Autodesk Fusion 360 part; units mm, degrees
sketch "Sketch1" plane through (0, 0, 0) normal (0, 0, 1) x (1, 0, 0)
  circle A0 centre (0, 0) radius 20
  line L0 (1, -19.975) -> (1, -21.1)
  line L1 (1, -21.1) -> (-1, -21.1)
  line L2 (-1, -21.1) -> (-1, -19.975)
  line L3 (18.7731, 9.684) -> (17.7988, 9.1215)
  line L4 (17.7731, 11.416) -> (18.7731, 9.684)
  line L5 (16.7988, 10.8535) -> (17.7731, 11.416)
  line L6 (-17.7731, 11.416) -> (-16.7988, 10.8535)
  line L7 (-18.7731, 9.684) -> (-17.7731, 11.416)
  line L8 (-17.7988, 9.1215) -> (-18.7731, 9.684)
  dimension "d5" = 40
  dimension "d9" = 2
  dimension "d12" = 360
extrude "Extrude2" add sketch "Sketch1" along normal blind 30 contours A0
shell "Shell2" thickness 1.5 removed faces 1 at (-4.9181, 4.3771, 30)
extrude "Extrude3" add sketch "Sketch1" along normal up to surface (30 mm away) contours A0 L3 L4 L5 | A0 L0 L1 L2 | A0 L6 L7 L8
The model under review builds one solid part; all positions refer to its coordinate system, in mm. A direction names the side the tool comes from. Give positions to 0.01 mm unless a question says otherwise; leave off trailing zeros. Loops run counter-clockwise (first coordinate to the right, second up) from the corner with the lowest first, then second, coordinate; pieces in that order, holes last. Notation, with made-up numbers: (-28.75, 18.25) -> (-12.75, 18.25) arc R22 cw to (-12.75, 55.25) -> close; hole circle Ø6 at (-19.5, 82). An arc over 180 degrees is marked (long way). Write each question's results on one line, items separated by ' | '.
1) Tool access review of faces 1 (the face through (17.28, 11.13, 14.79)), 2 (the face through (-18.28, 9.4, 14.79)), 3 (the face through (-4.01, 18.06, 15.55)), 4 (the face through (1, -20.5, 14.8)), 5 (the face through (-1, -20.5, 14.8)): name each direction out of +Z, -Z, +X, -X, +Y, -Y from which nothing blocks a thin tool from reaching the whole face with its end or side.
Conclusion:
face 1: +Z, -Z, +Y | face 2: +Z, -Z, -X | face 3: +Z | face 4: +Z, -Z, +X, -Y | face 5: +Z, -Z, -X, -Y
2) Draft analysis for pull direction X (two halves, no side actions). For faces 6 (the face through (-17.18, -10.24, 14.79)), 7 (the face through (0, 0, 1.5)), 8 (the face through (18.293, 9.407, 14.79)), state which applies: pulls with the +X half, pulls with the -X half, needs draft (parallel to the pull), parting line crosses it, or undercut.
Conclusion:
face 6: pulls with the -X half | face 7: undercut | face 8: pulls with the +X half
3) Take a section at A-A, the plane y = 0. Give the boundary of the cut face in (x, z).
Conclusion:
outline: (-20, 0) -> (20, 0) -> (20, 30) -> (18.5, 30) -> (18.5, 1.5) -> (-18.5, 1.5) -> (-18.5, 30) -> (-20, 30) -> close
4) Take a section at C-C, the plane z = 8. Give the boundary of the cut face in (x, y) (1 decimal), plus the area to 3 significant figures.
Conclusion:
outline: (-18.8, 9.7) -> (-17.8, 9.1) arc R20 ccw to (-1, -20) -> (-1, -21.1) -> (1, -21.1) -> (1, -20) arc R20 ccw to (17.8, 9.1) -> (18.8, 9.7) -> (17.8, 11.4) -> (16.8, 10.9) arc R20 ccw to (-16.8, 10.9) -> (-17.8, 11.4) -> close; hole circle Ø37 at (0, 0) | area: 188 mm^2
5) Insertion check: pin 1 Ø12 at (y, z) = (13, 17.5) entering from +X; pin 2 Ø2 at (x, z) = (-3, 8.5) entering from +Y; pin 3 Ø1 at (x, z) = (-2, 25) entering from -Y; pin 4 Ø8 at (x, y) = (1.5, 1) entering from -Z. Each pin has a flat end and moves straight along its axis. Give the tip position at first contact, or say it passes through.
Conclusion:
pin 1: stops at x = 18.77 | pin 2: stops at y = 19.9 | pin 3: stops at y = -19.94 | pin 4: stops at z = 0
6) Take a section at B-B, the plane x = 0. Give the boundary of the cut face in (y, z), plus the area to 4 significant figures.
Conclusion:
outline: (-21.1, 0) -> (20, 0) -> (20, 30) -> (18.5, 30) -> (18.5, 1.5) -> (-18.5, 1.5) -> (-18.5, 30) -> (-21.1, 30) -> close | area: 178.5 mm^2
7) For line 1 along Y through (x, z) = (0, 9); line 2 along X through (y, z) = (0, 18.25); line 3 along Z through (x, y) = (-13, -0.5), list the stretches that pass through material, from the lowest coordinate up. Write a range as from..to.
Conclusion:
line 1: y = -21.1..-18.5, 18.5..20 | line 2: x = -20..-18.5, 18.5..20 | line 3: z = 0..1.5
